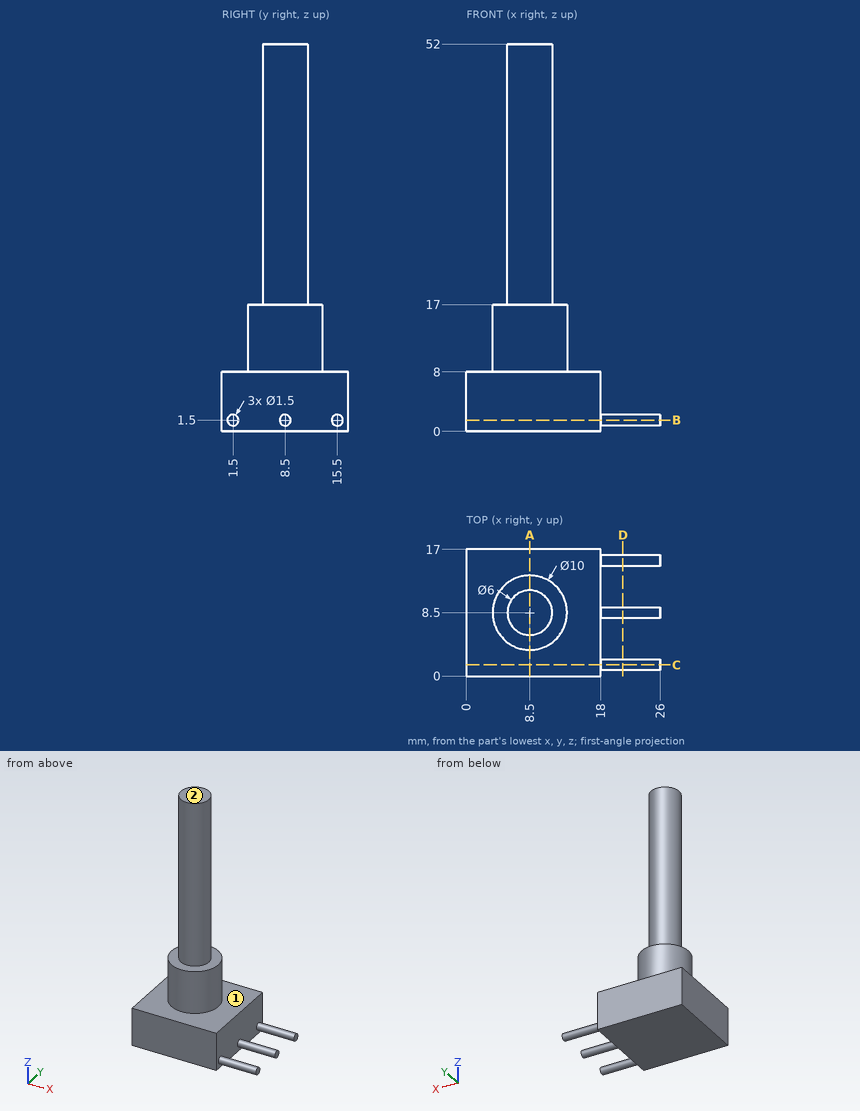
Design review of the part shown in the three views and the two pictorial views. Dimensions are in mm from the part's minimum x, y and z. A direction names the side the tool comes from. Coordinates: 2 decimals unless noted, no trailing zeros. Order: outer loops, then holes, each group sorted by start corner. A loop starts at its lowest first (then second) coordinate and runs counter-clockwise, first axis right, second up.
Item 1: For the marked faces 1 and 2, list the 3-axis set-ups (+Z, -Z, +X, -X, +Y, -Y) from which the entire face can be reached by the end or side of a thin tool; tool diameter is ignored.
Item 2: Take a section at A-A, the plane x = 8.5. Write out the cut boundary in (y, z).
Item 3: For line 1 (X direction, y = 4.5, z = 15.5); line 2 (X direction, y = 12.75, z = 2.5); line 3 (Y direction, x = 8.75, z = 41), list the stretches that pass through material, from the lowest coordinate up.
Item 4: For pin 1 Ø2 at (x, y) = (15.5, 11) entering from +Z; pin 2 Ø6.5 at (y, z) = (6.5, 4.5) entering from +X; pin 3 Ø2 at (y, z) = (12.5, 15.5) entering from -X; pin 4 Ø5 at (x, z) = (12, 30) entering from -Y, all flat-tipped, find the tip position at first contact; note any pin that passes through.
Item 5: Take a section at C-C, the plane y = 1.5. Write out the cut boundary in (x, z), then the cut area to 3 significant figures.
Item 6: Take a section at B-B, the plane z = 1.5. Write out the cut boundary in (x, y), then the cut area to 3 significant figures.
Item 7: Take a section at D-D, the plane x = 21. Write out the cut boundary in (y, z).
The answers:
1. face 1: +Z
1. face 2: +Z, +X, -X, +Y, -Y
2. outline: (0, 0) - (17, 0) - (17, 8) - (13.5, 8) - (13.5, 17) - (11.5, 17) - (11.5, 52) - (5.5, 52) - (5.5, 17) - (3.5, 17) - (3.5, 8) - (0, 8) - close
3. line 1: x = 5.5 to 11.5
3. line 2: x = 0 to 18
3. line 3: y = 5.51 to 11.49
4. pin 1: stops at z = 8
4. pin 2: stops at x = 26
4. pin 3: stops at x = 4.5
4. pin 4: stops at y = 5.67
5. outline: (0, 0) - (18, 0) - (18, 0.75) - (26, 0.75) - (26, 2.25) - (18, 2.25) - (18, 8) - (0, 8) - close
5. area: 156 mm2
6. outline: (0, 0) - (18, 0) - (18, 0.75) - (26, 0.75) - (26, 2.25) - (18, 2.25) - (18, 7.75) - (26, 7.75) - (26, 9.25) - (18, 9.25) - (18, 14.75) - (26, 14.75) - (26, 16.25) - (18, 16.25) - (18, 17) - (0, 17) - close
6. area: 342 mm2
7. outline: circle Ø1.5 at (1.5, 1.5); circle Ø1.5 at (8.5, 1.5); circle Ø1.5 at (15.5, 1.5)
